Geometry: see drawing. Coordinates: mm, zero at the bounding-box minimum. A direction names the side the tool comes from. Give positions to 0.01 mm unless a question says otherwise; leave off trailing zeros. Order: outer loops, then holes, each group sorted by start corner. A loop starts at its lowest first (then second) coordinate and runs counter-clockwise, first axis right, second up. Notation, with made-up numbers: M 77.5,43 L 99.5,43 A18 cw 99.5,48 Z; hole C -3,17.5 d5. An arc over 180 degrees is marked long. Use a Markdown table: item, result.
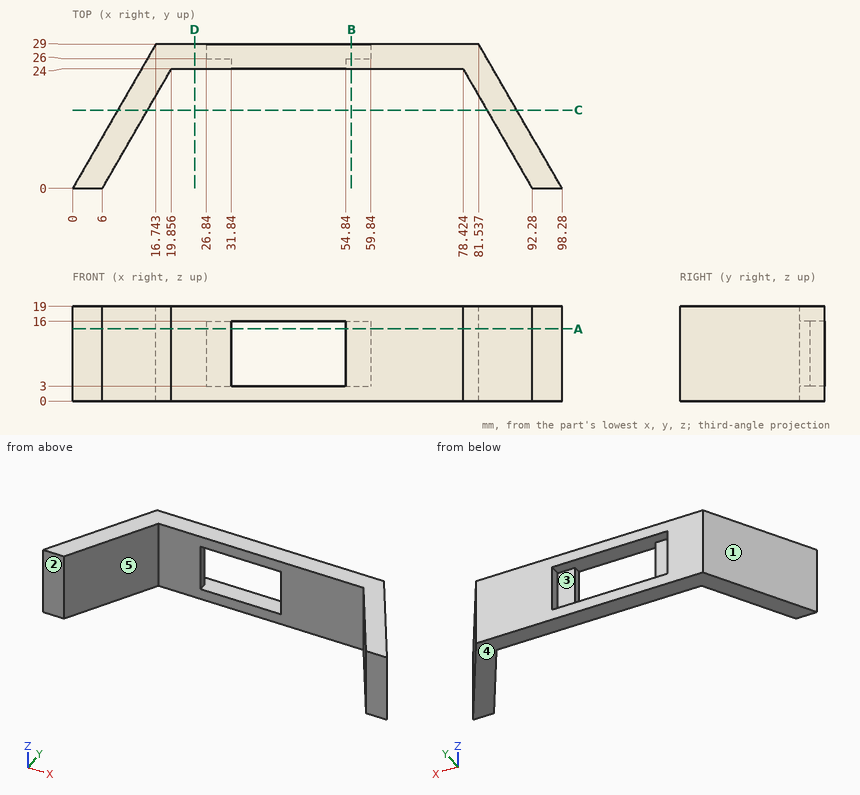
1) Cut plane A-A on z = 14.5. Return loops of the section in (x, y).
Response values:
| item | result |
|---|---|
| outline | M 0,0 L 6,0 L 19.86,24 L 31.84,24 L 31.84,26 L 26.84,26 L 26.84,29 L 16.74,29 Z; M 54.84,24 L 78.42,24 L 92.28,0 L 98.28,0 L 81.54,29 L 59.84,29 L 59.84,26 L 54.84,26 Z |
2) Mould query, pull axis X, two halves, no side actions, for the marked faces 1, 2 and 3. Classes: released by +X, released by -X, zero draft, split by the parting line, or undercut.
Response values:
| item | result |
|---|---|
| face 1 | released by -X |
| face 2 | zero draft |
| face 3 | undercut |
3) Cut plane B-B on x = 56. Return loops of the section in (y, z), and give its area (3 significant figures).
Response values:
| item | result |
|---|---|
| outline | M 24,0 L 29,0 L 29,3 L 26,3 L 26,16 L 29,16 L 29,19 L 24,19 Z |
| area | 56.0 mm² |
4) Reachability of the marked faces 4 and 5 from +Z, -Z, +X, -X, +Y, -Y: full face, straight path, thin tool, end or side. Return the list, or none.
Response values:
| item | result |
|---|---|
| face 4 | -Z, +X, -X, +Y, -Y |
| face 5 | +Z, -Z, -Y |
5) First-contact query: pin 1 Ø1.5 at (x, z) = (30, 6.5) entering from +Y; pin 2 Ø6 at (y, z) = (26, 13) entering from -X; pin 3 Ø1 at (y, z) = (25, 7) entering from +X (1 decimal). Flat tips, straight axial feed; report the tip coordinate or a pass-through.
Response values:
| item | result |
|---|---|
| pin 1 | stops at y = 26 |
| pin 2 | stops at x = 13.28 |
| pin 3 | stops at x = 84.1 |
6) Material intervals for line 1 (X direction, y = 22.25, z = 7.75) (1 decimal); line 2 (X direction, y = 14, z = 8.5); line 3 (Y direction, x = 67.5, z = 4.75), sorted ascending. Write a range as from..to.
Response values:
| item | result |
|---|---|
| line 1 | x = 12.8..18.8, 79.4..85.4 |
| line 2 | x = 8.08..14.08, 84.2..90.2 |
| line 3 | y = 24..29 |
7) Cut plane C-C on y = 15.75. Return loops of the section in (x, z), and give its area (3 significant figures).
Response values:
| item | result |
|---|---|
| outline | M 9.09,0 L 15.09,0 L 15.09,19 L 9.09,19 Z; M 83.19,0 L 89.19,0 L 89.19,19 L 83.19,19 Z |
| area | 228 mm² |
8) Cut plane D-D on x = 24.5. Return loops of the section in (y, z), and give its area (3 significant figures).
Response values:
| item | result |
|---|---|
| outline | M 24,0 L 29,0 L 29,19 L 24,19 Z |
| area | 95.0 mm² |
